Solid Edge part; units mm, degrees
sketch "Sketch1" plane through (0, 0, 0) normal (0, 0, 1) x (1, 0, 0)
  circle A0 centre (0, 0) radius 26.5
  circle A1 centre (0, 0) radius 34
extrude "Protrusion1" add sketch "Sketch1" along normal blind 3
sketch "Sketch2" plane through (0, 0, 3) normal (0, 0, 1) x (1, 0, 0)
  circle A0 centre (0, 0) radius 31.5
  circle A1 centre (0, 0) radius 34
extrude "ExtrudedProtrusion_2" add sketch "Sketch2" along normal blind 17
fillet "Round_1" radius 2 1 edges at (-34, 0, 0)
sketch "Sketch3" plane through (0, 0, 20) normal (0, 0, 1) x (1, 0, 0)
  line L0 (10, 32.4962) -> (10, 50)
  line L1 (-10, 50) -> (-10, 32.4962)
  arc A0 (-10, 32.4962) -> (10, 32.4962) centre (0, 0) cw
  arc A1 (-10, 50) -> (10, 50) centre (0, 50) cw
  circle A2 centre (0, 50) radius 3
  line L2 (50, 10) -> (32.4962, 10)
  arc A3 (32.4962, 10) -> (32.4962, -10) centre (0, 0) cw
  line L3 (32.4962, -10) -> (50, -10)
  arc A4 (50, 10) -> (50, -10) centre (50, 0) cw
  circle A5 centre (50, 0) radius 3
  circle A6 centre (0, -50) radius 3
  line L4 (-10, -32.4962) -> (-10, -50)
  line L5 (10, -50) -> (10, -32.4962)
  arc A7 (10, -50) -> (-10, -50) centre (0, -50) cw
  arc A8 (10, -32.4962) -> (-10, -32.4962) centre (0, 0) cw
  line L6 (-50, -10) -> (-32.4962, -10)
  arc A9 (-32.4962, -10) -> (-32.4962, 10) centre (0, 0) cw
  line L7 (-32.4962, 10) -> (-50, 10)
  arc A10 (-50, -10) -> (-50, 10) centre (-50, 0) cw
  circle A11 centre (-50, 0) radius 3
extrude "ExtrudedProtrusion_3" add sketch "Sketch3" against normal blind 5
fillet "Round_2" radius 2 4 edges at (34, 0, 15) (0, -34, 15) (-34, 0, 15) (0, 34, 15)
properties material "ABS, alto impacto"
Geometry check sheet. Reference: the model listing, model coordinates, mm. A direction names the side the tool comes from. Give positions to 0.01 mm unless a question says otherwise; leave off trailing zeros. Loops run counter-clockwise (first coordinate to the right, second up) from the corner with the lowest first, then second, coordinate; pieces in that order, holes last.
(1) Section check A-A on y = 0. Record the cut outline in (x, z), then the cut area to 3 significant figures.
From the geometry:
outline: (-60, 15) - (-53, 15) - (-53, 20) - (-60, 20) - close; (-47, 15) - (-36, 15) arc R2 cw to (-34, 13) - (-34, 2) arc R2 ccw to (-32, 0) - (-26.5, 0) - (-26.5, 3) - (-31.5, 3) - (-31.5, 20) - (-47, 20) - close; (26.5, 0) - (32, 0) arc R2 ccw to (34, 2) - (34, 13) arc R2 cw to (36, 15) - (47, 15) - (47, 20) - (31.5, 20) - (31.5, 3) - (26.5, 3) - close; (53, 15) - (60, 15) - (60, 20) - (53, 20) - close
area: 330 mm2
(2) Depth check by flat-ended pin: pin 1 Ø12 at (x, z) = (-26.5, 2.5) entering from +Y; pin 2 Ø10 at (x, y) = (-3.5, 44.5) entering from -Z; pin 3 Ø6 at (x, z) = (-33, 4.5) entering from -Y; pin 4 Ø5.5 at (x, y) = (0, -50) entering from -Z. Enter the tip coordinate at first touch or a pass-through.
From the geometry:
pin 1: stops at y = 27.12
pin 2: stops at z = 15
pin 3: stops at y = -16
pin 4: passes through
(3) Thickness scan on L1, parallel to Y at x = 0, z = 17.4; L2, parallel to Y at x = 50, z = 17.45; L3, parallel to Z at x = -6.5, y = -46.5. Record the ranges inside material, lowest first.
From the geometry:
L1: y = -60 to -53, -47 to -31.5, 31.5 to 47, 53 to 60
L2: y = -10 to -3, 3 to 10
L3: z = 15 to 20
(4) Section check D-D on y = -44. Record the cut outline in (x, z), then the cut area to 4 significant figures.
From the geometry:
outline: (-10, 15) - (10, 15) - (10, 20) - (-10, 20) - close
area: 100.0 mm2
(5) Section check C-C on z = 5.5. Record the cut outline in (x, y).
From the geometry:
outline: circle Ø68 at (0, 0); hole circle Ø63 at (0, 0)
(6) Set-up check for faces 1 (the flat face through (41, 10, 17)), 2 (the flat face through (-41, -10, 17)), 3 (the flat face through (-10, 41, 17)): record each of +Z, -Z, +X, -X, +Y, -Y from which the full face is reachable in a straight line by a thin tool's end or side.
From the geometry:
face 1: +Z, -Z, +X, +Y
face 2: +Z, -Z, -X, -Y
face 3: +Z, -Z, -X, +Y
(7) Release check for a two-part mould opening along X. For faces 4 (the flat face through (0, -44, 15)), 5 (the cylindrical face through (-4.101, -31.232, 11.381)), 6 (the flat face through (10, -41, 17)) record: released by +X, released by -X, zero draft, split by the parting line, or undercut.
From the geometry:
face 4: zero draft
face 5: undercut
face 6: released by +X
